Work out the finished part from the listing and answer in its coordinate system (mm). A direction names the side the tool comes from. Give positions to 0.01 mm unless a question says otherwise; leave off trailing zeros. Order: outer loops, then holes, each group sorted by start corner. A loop starts at its lowest first (then second) coordinate and runs counter-clockwise, first axis right, second up. Notation, with made-up numbers: (21.5, -21.5) - (40.5, -21.5) arc R23 ccw to (40.5, -5.5) - close; hole circle Ø5 at (14.5, 25). An arc over 180 degrees is marked (long way). Return JSON: item names as keys, results as strings. Group by question number.
from build123d import *

# Parameters (mm, degrees)
BOSS_EXTRUDE1_DEPTH = 3.7


with BuildPart() as part:
    # Model → Boss-Extrude1 (new body)
    with BuildSketch(Plane.XY):
        Polygon((-5.997220875, 216.82832197), (1.346e-06, 216.82832197), (1.346e-06, 220.814711934), (10.301111378, 220.814711934), (10.301111378, 216.82832197), (18.026945247, 216.82832197), (18.026945247, 220.814711934), (26.31722235, 220.814711934), (26.31722235, 216.82832197), (34.007778034, 216.82832197), (34.007778034, 220.814711934), (42.333333323, 220.814711934), (42.333333323, 216.82832197), (50.023888607, 216.82832197), (50.023888607, 220.814711934), (60.325001331, 220.814711934), (60.325001331, 216.82832197), (66.322223551, 216.82832197), (66.322223551, 210.831099749), (70.308610824, 210.831099749), (70.308610824, 200.529989717), (66.322223551, 200.529989717), (66.322223551, 192.80415652), (70.308610824, 192.80415652), (70.308610824, 184.513878576), (66.322223551, 184.513878576), (66.322223551, 176.823322787), (70.308610824, 176.823322787), (70.308610824, 168.533045011), (66.322223551, 168.533045011), (66.322223551, 160.807212487), (70.308610824, 160.807212487), (70.308610824, 150.506099764), (66.322223551, 150.506099764), (66.322223551, 144.508877543), (60.325001331, 144.508877543), (60.325001331, 140.522487579), (50.023888607, 140.522487579), (50.023888607, 144.508877543), (42.333333323, 144.508877543), (42.333333323, 140.522487579), (34.007778034, 140.522487579), (34.007778034, 144.508877543), (26.31722235, 144.508877543), (26.31722235, 140.522487579), (18.026945247, 140.522487579), (18.026945247, 144.508877543), (10.301111378, 144.508877543), (10.301111378, 140.522487579), (1.346e-06, 140.522487579), (1.346e-06, 144.508877543), (-5.997220875, 144.508877543), (-5.997220875, 150.506099764), (-9.983610839, 150.506099764), (-9.983610839, 160.807212487), (-5.997220875, 160.807212487), (-5.997220875, 168.533045011), (-9.983610839, 168.533045011), (-9.983610839, 176.823322787), (-5.997220875, 176.823322787), (-5.997220875, 184.513878576), (-9.983610839, 184.513878576), (-9.983610839, 192.80415652), (-5.997220875, 192.80415652), (-5.997220875, 200.529989717), (-9.983610839, 200.529989717), (-9.983610839, 210.831099749), (-5.997220875, 210.831099749), align=None)
        with BuildLine():
            add(Edge.make_bspline(
                [(4.409715492, 198.940379596), (3.805731041, 198.940379596), (3.316103574, 199.430003026), (3.316103574, 200.03399286), (3.316103574, 200.637982694), (3.805731041, 201.127606124), (4.409715492, 201.127606124)],
                knots=[2, 2, 2, 2, 3, 3, 3, 4, 4, 4, 4], degree=3))
            add(Edge.make_bspline(
                [(4.409715492, 201.127606124), (5.013699944, 201.127606124), (5.503326065, 200.637982694), (5.503326065, 200.03399286), (5.503326065, 199.430003026), (5.013699944, 198.940379596), (4.409715492, 198.940379596)],
                knots=[0, 0, 0, 0, 1, 1, 1, 2, 2, 2, 2], degree=3))
        make_face(mode=Mode.SUBTRACT)
        with BuildLine():
            add(Edge.make_bspline(
                [(55.915272381, 160.205373146), (55.31128793, 160.205373146), (54.821661808, 160.694996576), (54.821661808, 161.298986411), (54.821661808, 161.902976245), (55.31128793, 162.392599675), (55.915272381, 162.392599675)],
                knots=[2, 2, 2, 2, 3, 3, 3, 4, 4, 4, 4], degree=3))
            add(Edge.make_bspline(
                [(55.915272381, 162.392599675), (56.519256832, 162.392599675), (57.008882953, 161.902976245), (57.008882953, 161.298986411), (57.008882953, 160.694996576), (56.519256832, 160.205373146), (55.915272381, 160.205373146)],
                knots=[0, 0, 0, 0, 1, 1, 1, 2, 2, 2, 2], degree=3))
        make_face(mode=Mode.SUBTRACT)
        with BuildLine():
            add(Edge.make_bspline(
                [(4.409715492, 160.205373146), (3.805731041, 160.205373146), (3.316103574, 160.694996576), (3.316103574, 161.298986411), (3.316103574, 161.902976245), (3.805731041, 162.392599675), (4.409715492, 162.392599675)],
                knots=[2, 2, 2, 2, 3, 3, 3, 4, 4, 4, 4], degree=3))
            add(Edge.make_bspline(
                [(4.409715492, 162.392599675), (5.013699944, 162.392599675), (5.503326065, 161.902976245), (5.503326065, 161.298986411), (5.503326065, 160.694996576), (5.013699944, 160.205373146), (4.409715492, 160.205373146)],
                knots=[0, 0, 0, 0, 1, 1, 1, 2, 2, 2, 2], degree=3))
        make_face(mode=Mode.SUBTRACT)
        with BuildLine():
            add(Edge.make_bspline(
                [(55.915272381, 198.940379596), (55.31128793, 198.940379596), (54.821661808, 199.430003026), (54.821661808, 200.03399286), (54.821661808, 200.637982694), (55.31128793, 201.127606124), (55.915272381, 201.127606124)],
                knots=[2, 2, 2, 2, 3, 3, 3, 4, 4, 4, 4], degree=3))
            add(Edge.make_bspline(
                [(55.915272381, 201.127606124), (56.519256832, 201.127606124), (57.008882953, 200.637982694), (57.008882953, 200.03399286), (57.008882953, 199.430003026), (56.519256832, 198.940379596), (55.915272381, 198.940379596)],
                knots=[0, 0, 0, 0, 1, 1, 1, 2, 2, 2, 2], degree=3))
        make_face(mode=Mode.SUBTRACT)
    extrude(amount=BOSS_EXTRUDE1_DEPTH)


solid = part.part
1. The part is cut by section A-A (y = 181). Give the vertices of the cut face in (x, z).
2. The part is cut by section C-C (z = 1.35). State how many separate pieces and enclosed holes the cut face has, and give its area (3 significant figures).
3. Determine the mould class of faces 1 (the flat face through (68, 150.506, 2)), 2 (the flat face through (60.325, 219, 2)), 3 (the flat face through (-8, 168.533, 2)) for opening direction Y: released by +Y, released by -Y, zero draft, split by the parting line, or undercut.
4. Consider probe 1 along X at (y, z) = (162, 3); probe 2 along Y at (x, z) = (-4, 2.05); probe 3 along X at (y, z) = (211.5, 2.4). Determine where each line is inside the solid, lowest interval first. Write a range as from..to.
5. Each of these flat-tipped pins is pushed along its axis until it touches: pin 1 (1.1 mm diameter, centred on x = -8.5, z = 2.5, fed in from -Y); pin 2 (1.8 mm diameter, centred on y = 179.5, z = 1.5, fed in from -X); pin 3 (1.1 mm diameter, centred on x = 32, z = 2.5, fed in from +Y). Where does it stop, or does it pass through?
6. The part is cut by section B-B (x = 31). Give the vertices of the cut face in (y, z).
7. A tool of negligible diameter and unlimited length cuts with its end or side. For faces 4 (the flat face through (-8, 200.53, 2)), 5 (the flat face through (42.333, 219, 2)), 6 (the flat face through (68, 192.804, 2)), from which of +Z, -Z, +X, -X, +Y, -Y can it reach the whole face along a straight path? Write none if from no direction.
Answers:
{
 "1": {"outline": "(-6, 0) - (66.32, 0) - (66.32, 3.7) - (-6, 3.7) - close"},
 "2": {"separate pieces": "1", "enclosed holes": "4", "area": "5,810 mm^2"},
 "3": {"face 1": "released by -Y", "face 2": "zero draft", "face 3": "undercut"},
 "4": {"probe 1": "x = -6..3.57, 5.25..55.08, 56.75..66.32", "probe 2": "y = 144.51..216.83", "probe 3": "x = -6..66.32"},
 "5": {"pin 1": "stops at y = 150.51", "pin 2": "stops at x = -6", "pin 3": "stops at y = 216.83"},
 "6": {"outline": "(144.51, 0) - (216.83, 0) - (216.83, 3.7) - (144.51, 3.7) - close"},
 "7": {"face 4": "+Z, -Z, -X", "face 5": "+Z, -Z, +Y", "face 6": "+Z, -Z, +X"}
}
